Work out the finished part from the listing and answer in its coordinate system (mm). A direction names the side the tool comes from. Coordinates: 2 decimals unless noted, no trailing zeros. Loops run counter-clockwise (first coordinate to the right, second up) from the corner with the lowest first, then second, coordinate; pieces in that order, holes last. Notation, with made-up numbers: (-14.5, 16) - (1.5, 16) arc R18 ccw to (1.5, 26) - close; hole circle Ø1 at (-39.5, 70). An arc over 180 degrees is marked (long way). Write each question's results on one line, items separated by ' | '. Start each with the question number.
1. Each of these flat-tipped pins is pushed along its axis until it touches: P1, Ø1.2, axis at y = 9, z = -27.5, coming from the +X side; P2, Ø16, axis at x = 180, y = 50, coming from the +Z side; P3, Ø4.5, axis at y = 7.5, z = 26.5, coming from the +X side; P4, Ø1.5, axis at x = 145, z = -32, coming from the -Y side. Where does it stop, or does it pass through?
2. Determine the mould class of faces 4 (the cylindrical face through (66.849, 14.957, 0.61)), 5 (the cylindrical face through (113.146, 6.911, -19.062)), 6 (the flat face through (200, 96, 0)) for opening direction Y: released by +Y, released by -Y, zero draft, split by the parting line, or undercut.
3. Find the intervals of material crossed by line 1 along X through (y, z) = (50, 14.5); line 2 along Z through (x, y) = (211, 78); line 3 along Y through (x, z) = (180, 6), in increasing order. Write a range as [from, to].
4. A cutting plane is placed at A-A on y = 69. Determine the outline of the cut face in (x, z).
5. A cutting plane is placed at B-B on x = -14. Determine the outline of the cut face in (y, z).
6. Which of the six approach directions +Z, -Z, +X, -X, +Y, -Y give full straight-line access (tool end or side, diameter ignored) to faces 1 (the flat face through (210, 96, 20)), 2 (the flat face through (93, 6, -22)), 3 (the flat face through (-43, 105, -4))?
7. A cutting plane is placed at C-C on y = 129. Determine the outline of the cut face in (x, z).
from build123d import *

# Parameters (mm, degrees)
ESQUISSE1_W                  = 52.5
ESQUISSE1_H                  = 105
BOSS_EXTRU_1_DEPTH           = 52.5
ESQUISSE2_W                  = 40
ESQUISSE2_H                  = 40
ESQUISSE2_W_2                = 20
ESQUISSE2_H_2                = 20
BOSS_EXTRU_2_DEPTH           = 45.5
BOSS_EXTRU_2_DEPTH_BACK      = 105
ESQUISSE2_3_W                = 42.5
ESQUISSE2_3_H                = 85
ENL_V_MAT_EXTRU_1_DEPTH      = 106
ENL_V_START                  = -2.5
ENL_V_MAT_EXTRU_3_DEPTH      = 51
ENL_V_START_2                = 2.5
ENL_V_MAT_EXTRU_4_DEPTH      = 51
ESQUISSE1_6_R                = 5
ENL_V_MAT_EXTRU_5_DEPTH      = 53.5
ENL_V_MAT_EXTRU_5_DEPTH_BACK = 53.5
ENL_V_START_3                = -20
ESQUISSE1_7_W                = 20
ESQUISSE1_7_H                = 90.5
ENL_V_MAT_EXTRU_6_DEPTH      = 32.5
ENL_V_START_4                = 20
ESQUISSE1_8_W                = 20
ESQUISSE1_8_H                = 90.5
ENL_V_MAT_EXTRU_7_DEPTH      = 32.5


with BuildPart() as part:
    # Esquisse1 → Boss.-Extru.1 (new body, symmetric)
    with BuildSketch(Plane.XY):
        with Locations((-26.25, 52.5)):
            Rectangle(ESQUISSE1_W, ESQUISSE1_H)
    extrude(amount=BOSS_EXTRU_1_DEPTH, both=True)

    # Esquisse2 → Boss.-Extru.2 (add, two sides)
    with BuildSketch(Plane(origin=(0, 105, 0), x_dir=(1, 0, 0), z_dir=(0, 1, 0))) as boss_extru_2_sk:
        Polygon((210, 20), (52.5, 45.091911765), (52.5, -45.091911765), (210, -20), (190, -20), (190, 20), align=None)
        Polygon((6, 52.5), (0, 52.5), (0, 42.5), (42.5, 42.5), (42.5, -42.5), (0, -42.5), (0, -52.5), (6, -52.5), (52.5, -45.091911765), (52.5, 45.091911765), align=None)
        with Locations((210, 0)):
            Rectangle(ESQUISSE2_W, ESQUISSE2_H)
        with Locations((210, 0)):
            Rectangle(ESQUISSE2_W_2, ESQUISSE2_H_2, mode=Mode.SUBTRACT)
    extrude(amount=BOSS_EXTRU_2_DEPTH)
    extrude(boss_extru_2_sk.sketch, amount=-BOSS_EXTRU_2_DEPTH_BACK)

    # Esquisse2_3 → Enl_v. mat.-Extru.1 (cut, through all)
    with BuildSketch(Plane(origin=(0, 105, 0), x_dir=(1, 0, 0), z_dir=(0, 1, 0))):
        with Locations((-21.25, 0)):
            Rectangle(ESQUISSE2_3_W, ESQUISSE2_3_H)
        with Locations((21.25, 0)):
            Rectangle(ESQUISSE2_3_W, ESQUISSE2_3_H)
    extrude(amount=-ENL_V_MAT_EXTRU_1_DEPTH, mode=Mode.SUBTRACT)

    # Esquisse1_4 → Enl_v. mat.-Extru.3 (cut, through all)
    with BuildSketch(Plane.XY.offset(ENL_V_START)):
        with BuildLine():
            Line((52.5, 105), (52.5, 20))
            Line((52.5, 20), (67.5, 20))
            ThreePointArc((67.5, 20), (74.571067812, 17.071067812), (77.5, 10))
            Line((77.5, 10), (77.5, 6))
            Line((77.5, 6), (108.975092222, 6))
            ThreePointArc((108.975092222, 6), (113.20127484, 6.93692213), (116.635536654, 9.572123903))
            Line((116.635536654, 9.572123903), (144.204786201, 42.427876097))
            ThreePointArc((144.204786201, 42.427876097), (147.639048015, 45.06307787), (151.865230633, 46))
            Line((151.865230633, 46), (170, 46))
            Line((170, 46), (170, 50))
            ThreePointArc((170, 50), (172.928932188, 57.071067812), (180, 60))
            Line((180, 60), (190, 60))
            Line((190, 60), (190, 150.5))
            Line((190, 150.5), (178.849703137, 150.5))
            ThreePointArc((178.849703137, 150.5), (174.623520519, 149.56307787), (171.189258706, 146.927876097))
            Line((171.189258706, 146.927876097), (139.004961186, 108.572123903))
            ThreePointArc((139.004961186, 108.572123903), (135.570699372, 105.93692213), (131.344516755, 105))
            Line((131.344516755, 105), (52.5, 105))
        make_face()
    extrude(amount=-ENL_V_MAT_EXTRU_3_DEPTH, mode=Mode.SUBTRACT)

    # Esquisse1_5 → Enl_v. mat.-Extru.4 (cut, through all)
    with BuildSketch(Plane.XY.offset(ENL_V_START_2)):
        with BuildLine():
            Line((52.5, 105), (52.5, 20))
            Line((52.5, 20), (67.5, 20))
            ThreePointArc((67.5, 20), (74.571067812, 17.071067812), (77.5, 10))
            Line((77.5, 10), (77.5, 6))
            Line((77.5, 6), (108.975092222, 6))
            ThreePointArc((108.975092222, 6), (113.20127484, 6.93692213), (116.635536654, 9.572123903))
            Line((116.635536654, 9.572123903), (144.204786201, 42.427876097))
            ThreePointArc((144.204786201, 42.427876097), (147.639048015, 45.06307787), (151.865230633, 46))
            Line((151.865230633, 46), (170, 46))
            Line((170, 46), (170, 50))
            ThreePointArc((170, 50), (172.928932188, 57.071067812), (180, 60))
            Line((180, 60), (190, 60))
            Line((190, 60), (190, 150.5))
            Line((190, 150.5), (178.849703137, 150.5))
            ThreePointArc((178.849703137, 150.5), (174.623520519, 149.56307787), (171.189258706, 146.927876097))
            Line((171.189258706, 146.927876097), (139.004961186, 108.572123903))
            ThreePointArc((139.004961186, 108.572123903), (135.570699372, 105.93692213), (131.344516755, 105))
            Line((131.344516755, 105), (52.5, 105))
        make_face()
    extrude(amount=ENL_V_MAT_EXTRU_4_DEPTH, mode=Mode.SUBTRACT)

    # Esquisse1_6 → Enl_v. mat.-Extru.5 (cut, two sides)
    with BuildSketch(Plane.XY) as enl_v_mat_extru_5_sk:
        with BuildLine():
            Line((0, 105), (52.5, 105))
            Line((52.5, 105), (131.344516755, 105))
            ThreePointArc((131.344516755, 105), (135.570699372, 105.93692213), (139.004961186, 108.572123903))
            Line((139.004961186, 108.572123903), (171.189258706, 146.927876097))
            ThreePointArc((171.189258706, 146.927876097), (174.623520519, 149.56307787), (178.849703137, 150.5))
            Line((178.849703137, 150.5), (0, 150.5))
            Line((0, 150.5), (0, 105))
        make_face()
        with BuildLine():
            ThreePointArc((119.433382603, 3.572123903), (115.999120789, 0.93692213), (111.772938171, 0))
            Line((111.772938171, 0), (230, 0))
            Line((230, 0), (230, 40))
            Line((230, 40), (210, 40))
            Line((210, 40), (154.663076582, 40))
            ThreePointArc((154.663076582, 40), (150.436893964, 39.06307787), (147.00263215, 36.427876097))
            Line((147.00263215, 36.427876097), (119.433382603, 3.572123903))
        make_face()
        with Locations((67.5, 10)):
            Circle(ESQUISSE1_6_R)
        with Locations((180, 50)):
            Circle(ESQUISSE1_6_R)
    extrude(amount=ENL_V_MAT_EXTRU_5_DEPTH, mode=Mode.SUBTRACT)
    extrude(enl_v_mat_extru_5_sk.sketch, amount=-ENL_V_MAT_EXTRU_5_DEPTH_BACK, mode=Mode.SUBTRACT)

    # Esquisse1_7 → Enl_v. mat.-Extru.6 (cut)
    with BuildSketch(Plane.XY.offset(ENL_V_START_3)):
        with Locations((200, 105.25)):
            Rectangle(ESQUISSE1_7_W, ESQUISSE1_7_H)
    extrude(amount=-ENL_V_MAT_EXTRU_6_DEPTH, mode=Mode.SUBTRACT)

    # Esquisse1_8 → Enl_v. mat.-Extru.7 (cut)
    with BuildSketch(Plane.XY.offset(ENL_V_START_4)):
        with Locations((200, 105.25)):
            Rectangle(ESQUISSE1_8_W, ESQUISSE1_8_H)
    extrude(amount=ENL_V_MAT_EXTRU_7_DEPTH, mode=Mode.SUBTRACT)


solid = part.part
Values:
1) P1: x = 124.49 | P2: z = 26.05 | P3: x = 124.62 | P4: through
2) face 4: undercut | face 5: released by +Y | face 6: zero draft
3) line 1: [-52.5, -42.5], [42.5, 52.5], [170, 175], [185, 230] | line 2: [-20, -10], [10, 20] | line 3: [40, 45], [55, 60]
4) outline: (-52.5, -52.5) - (6, -52.5) - (52.5, -45.09) - (52.5, -2.5) - (190, -2.5) - (190, -20) - (230, -20) - (230, 20) - (190, 20) - (190, 2.5) - (52.5, 2.5) - (52.5, 45.09) - (6, 52.5) - (-52.5, 52.5) - close; hole (-42.5, -42.5) - (42.5, -42.5) - (42.5, 42.5) - (-42.5, 42.5) - close; hole (200, -10) - (220, -10) - (220, 10) - (200, 10) - close
5) outline: (0, -52.5) - (105, -52.5) - (105, -42.5) - (0, -42.5) - close; (0, 42.5) - (105, 42.5) - (105, 52.5) - (0, 52.5) - close
6) face 1: +Z, +X, +Y | face 2: -Z, +Y | face 3: +Z, -Z, -X, +Y
7) outline: (156.15, -2.5) - (190, -2.5) - (190, -20) - (230, -20) - (230, 20) - (190, 20) - (190, 2.5) - (156.15, 2.5) - close; hole (200, -10) - (220, -10) - (220, 10) - (200, 10) - close
